Geometry: see drawing. Coordinates: mm, zero at the bounding-box minimum. Coordinates: 2 decimals unless noted, no trailing zeros. Order: outer loops, then holes, each group sorted by start corner. A loop starts at its lowest first (then second) coordinate and runs counter-clockwise, first axis right, second up. Notation, with made-up numbers: M 83,-36.75 L 123,-36.75 A9 ccw 123,-24.75 Z; hole C 1,61.5 d5. An arc over 180 degrees is marked long. Answer in a Markdown table with one row per item.
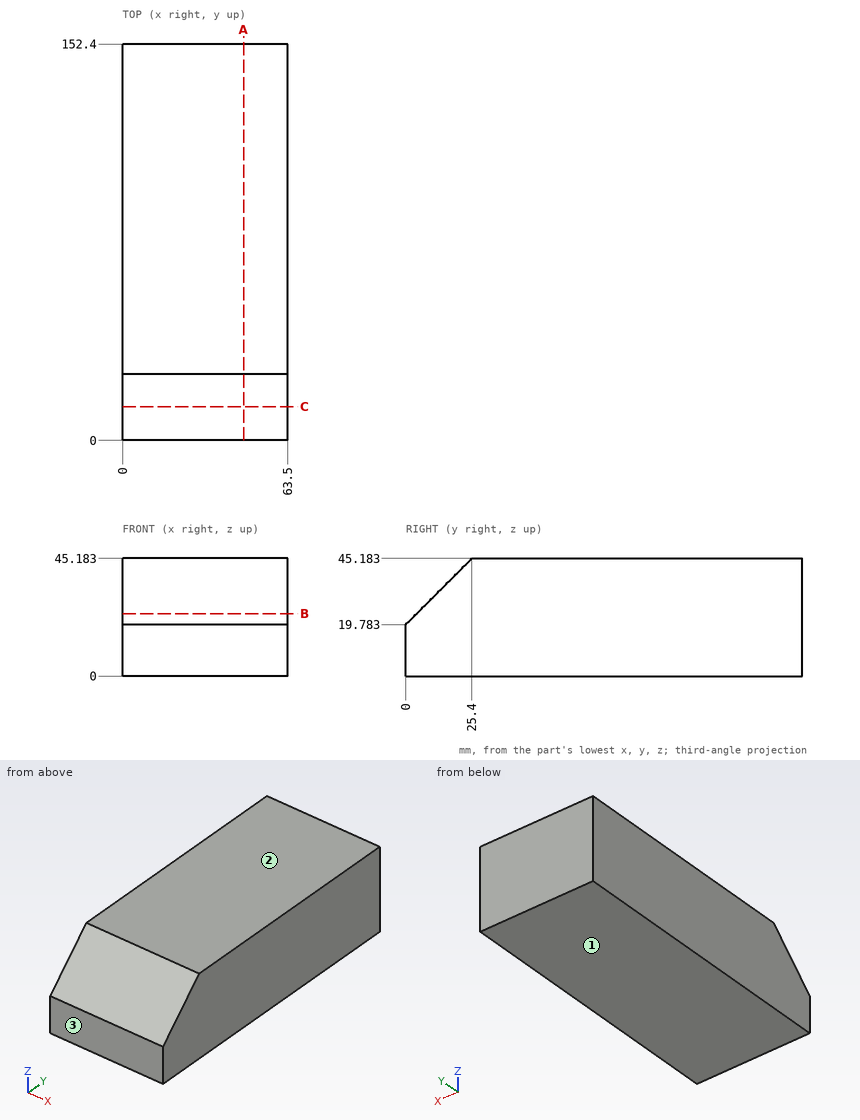
1) Material intervals for probe 1 along Y at (x, z) = (31, 28); probe 2 along Y at (x, z) = (26.5, 27); probe 3 along Z at (x, y) = (52.5, 16), sorted ascending.
Resolved:
| item | result |
|---|---|
| probe 1 | y = 8.22 to 152.4 |
| probe 2 | y = 7.22 to 152.4 |
| probe 3 | z = 0 to 35.78 |
2) Mould query, pull axis Z, two halves, no side actions, for the marked faces 1, 2 and 3. Classes: +Z half, -Z half, draft (parallel to the pull), parting line (faces both ways), or undercut.
Resolved:
| item | result |
|---|---|
| face 1 | -Z half |
| face 2 | +Z half |
| face 3 | draft |
3) Cut plane C-C, the plane y = 13. Output: boundary loops of the cut face in (x, z), and give its area (3 significant figures).
Resolved:
| item | result |
|---|---|
| outline | M 0,0 L 63.5,0 L 63.5,32.78 L 0,32.78 Z |
| area | 2,080 mm2 |
4) Cut plane A-A, the plane x = 46.5. Output: boundary loops of the cut face in (y, z).
Resolved:
| item | result |
|---|---|
| outline | M 0,0 L 152.4,0 L 152.4,45.18 L 25.4,45.18 L 0,19.78 Z |
5) Cut plane B-B, the plane z = 24. Output: boundary loops of the cut face in (x, y).
Resolved:
| item | result |
|---|---|
| outline | M 0,4.22 L 63.5,4.22 L 63.5,152.4 L 0,152.4 Z |
